Job drawing, mm, ordinate dimensions from the low corner. One solid piece. Coordinates: 2 decimals unless noted, no trailing zeros. Loops run counter-clockwise (first coordinate to the right, second up) from the corner with the lowest first, then second, coordinate; pieces in that order, holes last. Notation, with made-up numbers: (-17.5, 16) - (16.5, 16) arc R16 cw to (16.5, 33) - close; hole circle Ø9 at (54.5, -17.5). An arc over 180 degrees is marked (long way). Use a Markdown table: item, result. Add a question column.
1) Band-saw the part on D-D (y = 13.75). Give the cut face in (x, z), plus the area to 3 significant figures.
2) Pull direction Y, two halves, no side cores. Call the marked faces 1, 2, 3 and 4: +Y half, -Y half, draft (parallel to the pull), parting line (faces both ways), or undercut.
3) Probe probe 1 along Y at (x, z) = (9.9, 2.7); probe 2 along Y at (x, z) = (9.9, 38); probe 3 along Z at (x, y) = (7, 12.5). List the from-to ranges inside material, lowest first. Write a range as [from, to].
4) Band-saw the part on C-C (z = 9). Give the cut face in (x, y).
5) Drop flat-ended pins along their axis: P1, Ø1.5, axis at y = 15, z = 47.5, coming from the -X side; P2, Ø5, axis at x = 3, y = 6, coming from the -Z side; P3, Ø3, axis at y = 12.5, z = 39.5, coming from the +X side; P4, Ø10.5, axis at x = 9.9, y = 9.9, coming from the +Z side. Give the stop position or say it passes through.
6) Band-saw the part on A-A (y = 9.9). Give the cut face in (x, z).
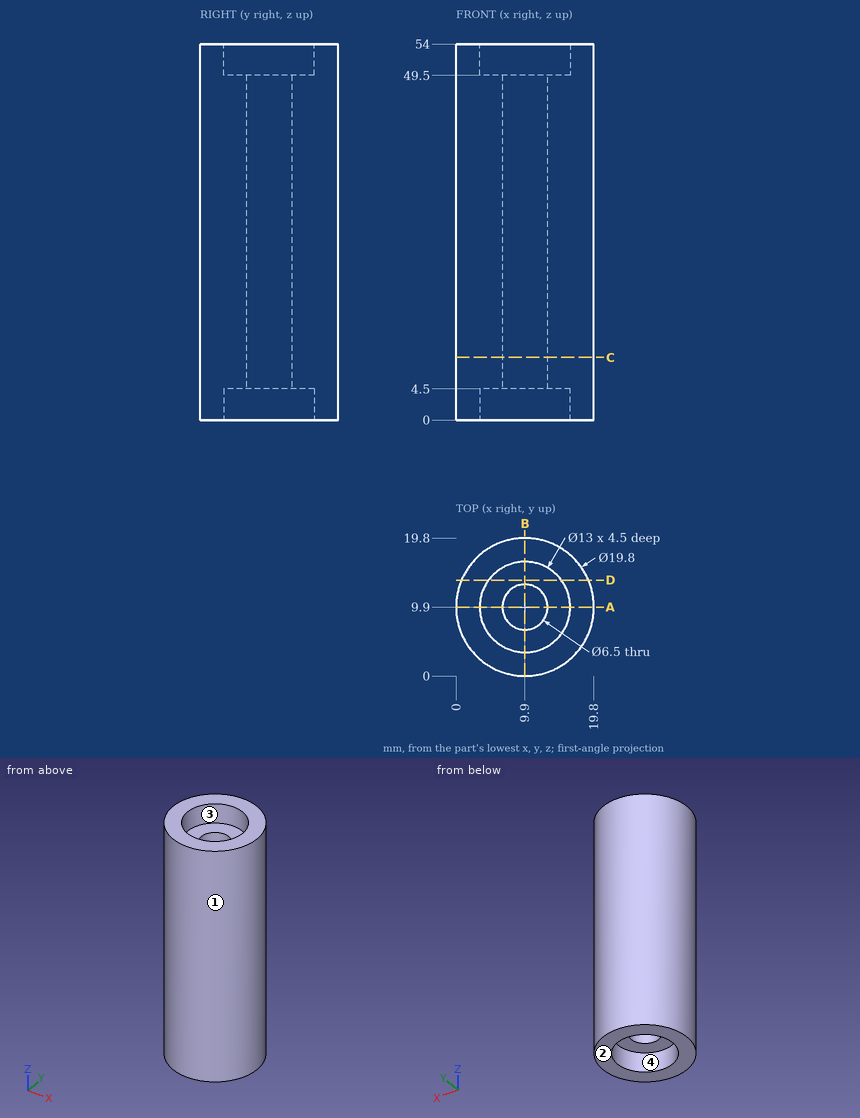
Answer block:
| question | item | result |
|---|---|---|
| 1 | outline | (0.78, 0) - (4.66, 0) - (4.66, 4.5) - (15.14, 4.5) - (15.14, 0) - (19.02, 0) - (19.02, 54) - (15.14, 54) - (15.14, 49.5) - (4.66, 49.5) - (4.66, 54) - (0.78, 54) - close |
| 1 | area | 891 mm2 |
| 2 | face 1 | parting line |
| 2 | face 2 | draft |
| 2 | face 3 | undercut |
| 2 | face 4 | undercut |
| 3 | probe 1 | [0, 3.4], [16.4, 19.8] |
| 3 | probe 2 | [0, 6.65], [13.15, 19.8] |
| 3 | probe 3 | [4.5, 49.5] |
| 4 | outline | circle Ø19.8 at (9.9, 9.9); hole circle Ø6.5 at (9.9, 9.9) |
| 5 | P1 | x = 1.01 |
| 5 | P2 | z = 0 |
| 5 | P3 | x = 19.74 |
| 5 | P4 | z = 49.5 |
| 6 | outline | (0, 0) - (3.4, 0) - (3.4, 4.5) - (6.65, 4.5) - (6.65, 49.5) - (3.4, 49.5) - (3.4, 54) - (0, 54) - close; (13.15, 4.5) - (16.4, 4.5) - (16.4, 0) - (19.8, 0) - (19.8, 54) - (16.4, 54) - (16.4, 49.5) - (13.15, 49.5) - close |
